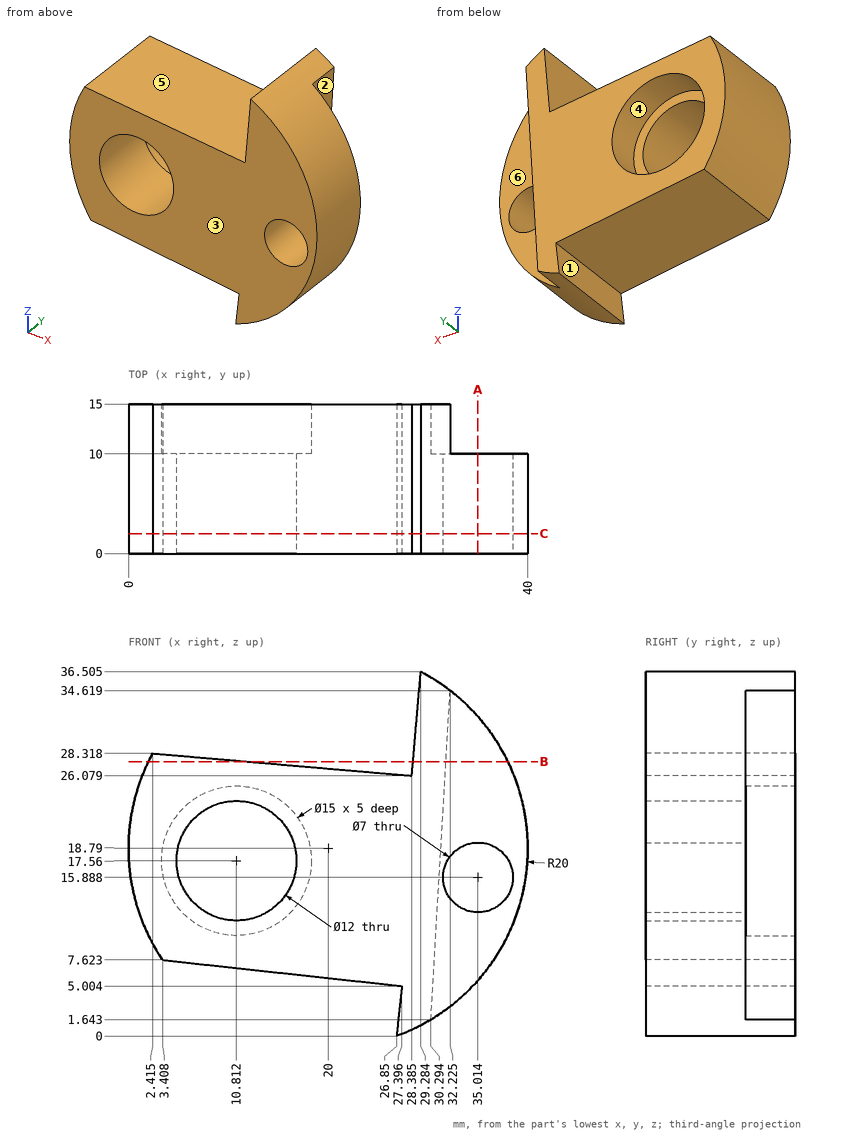
Could you check a few things on this drawing? It's one solid part, dimensions in mm from its lowest x, y, z. A direction names the side the tool comes from. Coordinates: 2 decimals unless noted, no trailing zeros. Write each loop counter-clockwise with the first axis right and the second up, starting at its lowest first coordinate (ties: lowest second). Pieces come first, ordered by that corner, then holes.
1) If we section it at B-B (z = 27.5): List the corners of the cut face in (x, y) for me (1 decimal).
Filled in:
outline: (2, 0) - (11.9, 0) - (11.9, 15) - (2, 15) - close; (28.5, 0) - (38, 0) - (38, 10) - (31.8, 10) - (31.8, 15) - (28.5, 15) - close
2) Thinking about a two-plate mould opening in Z: for the marked faces 1, 2 and 3, which applies, +Z half, -Z half, draft (parallel to the pull), parting line (faces both ways), or undercut?
Filled in:
face 1: undercut
face 2: -Z half
face 3: draft
3) Which directions (+Z, -Z, +X, -X, +Y, -Y) give clear straight access to the entire face, cutting with the end or side of a thin tool? Please do the marked faces 4, 5 and 6.
Filled in:
face 4: +Y
face 5: +Z, +Y, -Y
face 6: -Z, +X, +Y
4) If I drill on line 1 (Z direction, x = 34, y = 3.25) (1 decimal); line 2 (Z direction, x = 33.5, y = 4.25) (1 decimal); line 3 (X direction, y = 4.25, z = 20) (1 decimal), over which ranges is the centre line in solid material (lowest first)?
Filled in:
line 1: z = 4.5 to 12.5, 19.2 to 33.1
line 2: z = 4 to 12.7, 19 to 33.5
line 3: x = 0 to 5.3, 16.3 to 40
5) If we section it at C-C (y = 2): Count the separate pieces of the cut face and the enclosed holes in it, plus the area to 3 significant figures.
Filled in:
separate pieces: 1
enclosed holes: 2
area: 725 mm2
6) If we section it at A-A (x = 35): List the corners of the cut face in (y, z) for me.
Filled in:
outline: (0, 5.56) - (10, 5.56) - (10, 12.39) - (0, 12.39) - close; (0, 19.39) - (10, 19.39) - (10, 32.02) - (0, 32.02) - close
7) I'm going to push flat-ended pins straight in: pin 1 (6 mm diameter, centred on x = 4.5, y = 5, fed in from -Z); pin 2 (8 mm diameter, centred on x = 36.5, z = 19, fed in from +Y); pin 3 (8 mm diameter, centred on x = 22.5, y = 7.5, fed in from +Z); pin 4 (1 mm diameter, centred on x = 33, z = 14, fed in from +Y). Where does each tip first touch, or does it pass through?
Filled in:
pin 1: stops at z = 7.18
pin 2: stops at y = 10
pin 3: stops at z = 26.93
pin 4: passes through
